Autodesk Inventor part; units mm, degrees
ref_plane "YZ Plane" through (0, 0, 0) normal (1, 0, 0) x (0, 1, 0)
ref_plane "XZ Plane" through (0, 0, 0) normal (0, 1, 0) x (-1, 0, 0)
ref_plane "XY Plane" through (0, 0, 0) normal (0, 0, 1) x (1, 0, 0)
sketch "Skizze1" plane through (0, 0, 0) normal (0, 0, 1) x (1, 0, 0)
  line L0 (-7, 25) -> (0, 25)
  line L1 (0, 25) -> (0, -25)
  line L2 (0, -25) -> (-7, -25)
  line L3 (-7, -25) -> (-7, 25)
  point P0 (0, 0)
  point P1 (0, 0)
  dimension "d0" = 7
  dimension "d1" = 50
extrude "Extrusion1" add sketch "Skizze1" along normal blind 12
sketch "Skizze2" plane through (0, -25, 0) normal (1, 0, 0) x (0, 0, -1)
  line L0 (-10, 33) -> (0, 33)
  line L1 (0, 33) -> (0, 17)
  line L2 (0, 17) -> (-10, 17)
  line L3 (-10, 17) -> (-10, 33)
  line L4 (0, 0) -> (0, 50)
  line L5 (-12, 0) -> (-12, 50)
  point P0 (0, 25)
  point P1 (0, 25)
  point P2 (0, 25)
  dimension "d4" = 0
  dimension "d6" = 16
  dimension "d48" = 10
extrude "Extrusion2" add sketch "Skizze2" along normal blind 12
sketch "Skizze5" plane through (0, 0, 12) normal (0, 0, 1) x (1, 0, 0)
  line L0 (12, -3.525) -> (0, -3.525)
  line L1 (0, -3.525) -> (0, 3.525)
  line L2 (0, 3.525) -> (12, 3.525)
  line L3 (12, 3.525) -> (12, -3.525)
  line L4 (12, -3.525) -> (0, 3.525) construction
  line L5 (0, -3.525) -> (12, 3.525) construction
  line L6 (12, 8) -> (12, -8)
  point P0 (0, 0)
  point P1 (6, 0)
  point P2 (6, 0)
  point P3 (0, 0)
  point P4 (6, 0)
  dimension "d27" = 7.05
extrude "Extrusion3" cut sketch "Skizze5" against normal through all
sketch "Skizze6" plane through (0, 8, 12) normal (0, 1, 0) x (1, 0, 0)
  line L0 (0, 2) -> (0, 12) construction
  line L1 (0, 2) -> (12, 2) construction
  line L2 (12, 12) -> (12, 2) construction
  line L3 (0, 12) -> (12, 12) construction
  point P0 (0, 12)
  point P1 (8, 7)
  point P2 (12, 7)
  point P3 (6, 2)
  dimension "d38" = 8
  dimension "d47" = 5
hole "Bohrung3" at (8, 8, 5) direction (0, -1, 0) diameter 4.2 end through all
sketch "Skizze7" plane through (0, -3.525, 12) normal (1, 0, 0) x (0, 0, -1)
  line L0 (12, 7.05) -> (12, 0) construction
  line L1 (2, 7.05) -> (12, 7.05) construction
  line L2 (0, -21.475) -> (0, 28.525) construction
  line L3 (2, 0) -> (12, 0) construction
  line L4 (12, 0) -> (2, 0)
  line L5 (12, -21.475) -> (0, -21.475)
  line L6 (12, -21.475) -> (12, -4.475)
  line L7 (12, -4.475) -> (2, -4.475)
  line L8 (2, -4.475) -> (2, 0)
  line L9 (2, 7.05) -> (2, 11.525)
  line L10 (2, 11.525) -> (12, 11.525)
  line L11 (12, 11.525) -> (12, 28.525)
  line L12 (12, 28.525) -> (0, 28.525)
  line L13 (2, 7.05) -> (12, 7.05)
  point P0 (12, 3.525)
  point P1 (0, 0)
  point P2 (7, 3.525)
  point P3 (7, 0)
  point P4 (0, 3.525)
  point P5 (7, 7.05)
hole "Bohrung4" at (0, 0, 5) direction (-1, 0, 0) diameter 4.2 end through all
sketch "Skizze9" plane through (0, 0, 12) normal (0, 0, 1) x (1, 0, 0)
  line L0 (-7, -25) -> (0, -25)
  line L1 (0, -25) -> (0, 25)
  line L2 (0, 25) -> (-7, 25)
  line L3 (-7, 25) -> (-7, -25)
  arc A0 (-5.7446, -25) -> (-5.7446, 25) centre (-184, 0) ccw
  line L4 (0, -8) -> (12, -8)
  line L5 (-4, 0) -> (0, 0) construction
  line L6 (-2.2446, 25) -> (0, 16)
  line L7 (0, 8) -> (12, 8)
  line L8 (0, -16) -> (-2.2446, -25)
  point P0 (0, 0)
  dimension "d55" = 4
  dimension "d56" = 180
  dimension "d57" = 8
  dimension "d58" = 3.5
  dimension "d59" = 8
  dimension "d60" = 3.5
extrude "Extrusion4" cut sketch "Skizze9" against normal through all contours L3 L2 A0 L0 | L8 L1 L0 | L2 L1 L6
chamfer "Fase1" distance 0.5 angle 45 1 edges at (0, 0, 7.1)
properties part number "Schaufel_newtest" material "Aluminium 6061"
Here's how the part is built. I have some questions about the finished solid (model axes, mm). A direction names the side the tool comes from. Give positions to 0.01 mm unless a question says otherwise; leave off trailing zeros. Write each loop counter-clockwise with the first axis right and the second up, starting at its lowest first coordinate (ties: lowest second). Pieces come first, ordered by that corner, then holes.
(1) Imagine slicing it at B-B, the plane z = 5. Write out the boundary of the cut face in (x, y) (3 decimals), and give its area (3 significant figures).
Output values:
outline: (-5.745, -25) - (-2.245, -25) - (0, -16) - (0, -8) - (5.9, -8) - (5.9, -3.525) - (0, -3.525) - (0, -2.6) - (-0.5, -2.1) - (-4.012, -2.1) arc R180 cw to start; (-5.745, 25) arc R180 cw to (-4.012, 2.1) - (-0.5, 2.1) - (0, 2.6) - (0, 3.525) - (5.9, 3.525) - (5.9, 8) - (0, 8) - (0, 16) - (-2.245, 25) - close; (10.1, -8) - (12, -8) - (12, -3.525) - (10.1, -3.525) - close; (10.1, 3.525) - (12, 3.525) - (12, 8) - (10.1, 8) - close
area: 262 mm2
(2) Will these pins go through, and if not, where does the flat tip stop? pin 1 (2.5 mm diameter, centred on x = 8, z = 5, fed in from -Y); pin 2 (5 mm diameter, centred on x = 5, z = 3.5, fed in from -Y); pin 3 (4 mm diameter, centred on y = -18.5, z = 1, fed in from +X); pin 4 (2 mm diameter, centred on x = 8.5, y = 5.5, fed in from +Z).
Output values:
pin 1: passes through
pin 2: stops at y = -8
pin 3: stops at x = -0.12
pin 4: stops at z = 10
(3) Thinking about a two-plate mould opening in X: for faces 4 (the face through (5.918, -5.794, 4.727)), 5 (the face through (12, -6, 5)), 6 (the face through (-2.28, 2.05, 5.46)), which applies, pulls with the +X half, pulls with the -X half, needs draft (parallel to the pull), parting line crosses it, or undercut?
Output values:
face 4: undercut
face 5: pulls with the +X half
face 6: needs draft
(4) On a 3-axis mill with a long thin cutter (end or side, diameter ignored), from which of +Z, -Z, +X, -X, +Y, -Y can I reach the whole of each face in a straight line? I mean faces 1 (the face through (5, -3.525, 5)), 2 (the face through (5, -8, 5)), 3 (the face through (5, 8, 5)). Say none if no direction works.
Output values:
face 1: +Z, -Z, +X
face 2: +Z, -Z, +X, -Y
face 3: +Z, -Z, +X, +Y
(5) Imagine slicing it at D-D, the plane x = 8. Write out the boundary of the cut face in (y, z) (3 decimals), and give its area (3 significant figures).
Output values:
outline: (-8, 0) - (-3.525, 0) - (-3.525, 2.9) - (-8, 2.9) - close; (-8, 7.1) - (-3.525, 7.1) - (-3.525, 10) - (-8, 10) - close; (3.525, 0) - (8, 0) - (8, 2.9) - (3.525, 2.9) - close; (3.525, 7.1) - (8, 7.1) - (8, 10) - (3.525, 10) - close
area: 51.9 mm2
(6) If I drill on L1, parallel to Y at x = 2.75, z = 3.75 (3 decimals); L2, parallel to Z at x = -1.2, y = 0; L3, parallel to Z at x = 8, y = -5, over which ranges is the centre line in solid material (lowest first)?
Output values:
L1: y = -8 to -3.525, 3.525 to 8
L2: z = 0 to 2.9, 7.1 to 12
L3: z = 0 to 2.9, 7.1 to 10
(7) Imagine slicing it at C-C, the plane y = 0. Write out the boundary of the cut face in (x, z), and give its area (3 significant figures).
Output values:
outline: (-4, 0) - (0, 0) - (0, 2.4) - (-0.5, 2.9) - (-4, 2.9) - close; (-4, 7.1) - (-0.5, 7.1) - (0, 7.6) - (0, 12) - (-4, 12) - close
area: 31.0 mm2
(8) Imagine slicing it at A-A, the plane x = 3.5. Write out the boundary of the cut face in (y, z) (3 decimals), and give its area (3 significant figures).
Output values:
outline: (-8, 0) - (-3.525, 0) - (-3.525, 10) - (-8, 10) - close; (3.525, 0) - (8, 0) - (8, 10) - (3.525, 10) - close
area: 89.5 mm2
